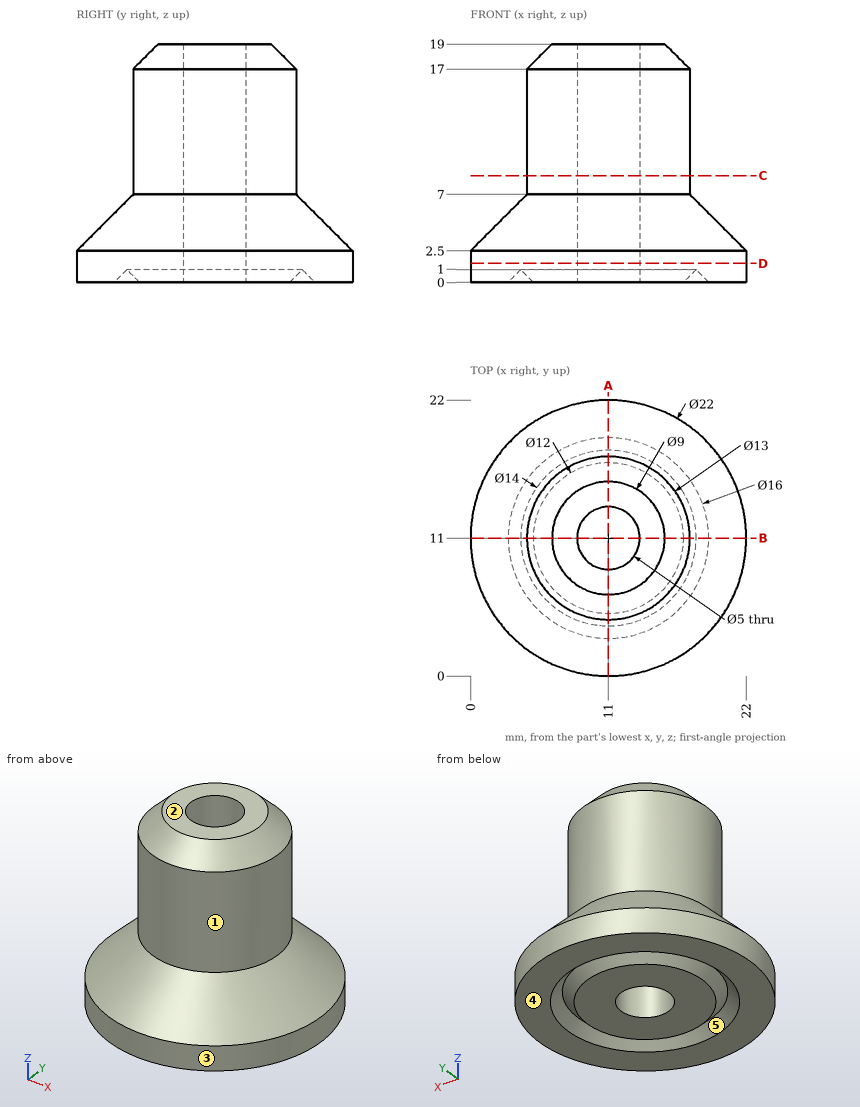
Job drawing, mm, ordinate dimensions from the low corner. One solid piece. A direction names the side the tool comes from. Coordinates: 2 decimals unless noted, no trailing zeros. Order: outer loops, then holes, each group sorted by start corner. A loop starts at its lowest first (then second) coordinate and runs counter-clockwise, first axis right, second up. Notation, with made-up numbers: (23, 14) -> (71, 14) arc R8 ccw to (71, 18) -> close; hole circle Ø7 at (63.25, 3.25). An arc over 180 degrees is marked (long way). Put each result on its own line as item: value. Start each with the question number.
(1) Probe line 1 along Y through (x, z) = (11, 10.75); line 2 along Y through (x, z) = (11, 4.5). List the from-to ranges inside material, lowest first. Write a range as [from, to].
(2) Band-saw the part on C-C (z = 8.5). Give the cut face in (x, y).
(3) Mould opens along X. For the marked faces 3, 4 and 5 say: pulls with the +X half, pulls with the -X half, needs draft (parallel to the pull), parting line crosses it, or undercut.
(4) Band-saw the part on D-D (z = 1.5). Give the cut face in (x, y), then the cut area to 3 significant figures.
(5) Band-saw the part on A-A (x = 11). Give the cut face in (y, z).
(6) Which spindle directions (+Z, -Z, +X, -X, +Y, -Y) get a long thin tool onto all of the face, cutting with end or side? Do the marked faces 1 and 2. Say none if no direction does.
(7) Pin check, flat tips, straight feed: pin 1 Ø5 at (y, z) = (14, 12) entering from +X; pin 2 Ø10 at (x, z) = (16.5, 7.5) entering from +Y; pin 3 Ø1 at (x, y) = (6, 10) entering from +Z. Stop position of each tip, or through.
Determined:
1. line 1: y = [4.5, 8.5], [13.5, 17.5]
1. line 2: y = [2, 8.5], [13.5, 20]
2. outline: circle Ø13 at (11, 11); hole circle Ø5 at (11, 11)
3. face 3: parting line crosses it
3. face 4: needs draft
3. face 5: undercut
4. outline: circle Ø22 at (11, 11); hole circle Ø5 at (11, 11)
4. area: 360 mm²
5. outline: (0, 0) -> (3, 0) -> (4, 1) -> (5, 0) -> (8.5, 0) -> (8.5, 19) -> (6.5, 19) -> (4.5, 17) -> (4.5, 7) -> (0, 2.5) -> close; (13.5, 0) -> (17, 0) -> (18, 1) -> (19, 0) -> (22, 0) -> (22, 2.5) -> (17.5, 7) -> (17.5, 17) -> (15.5, 19) -> (13.5, 19) -> close
6. face 1: +Z
6. face 2: +Z, +X, -X, +Y, -Y
7. pin 1: stops at x = 17.48
7. pin 2: stops at y = 21
7. pin 3: stops at z = 18.9
